The model under review builds one solid part; all positions refer to its coordinate system, in mm. Coordinates: 2 decimals unless noted, no trailing zeros. Loops run counter-clockwise (first coordinate to the right, second up) from the corner with the lowest first, then second, coordinate; pieces in that order, holes last. Notation, with made-up numbers: (-34.5, 10.5) - (-3.5, 10.5) arc R27 cw to (-3.5, 30.5) - close; hole circle Ø11 at (63.5, -24). An arc over 180 degrees is marked (long way). Answer in a Markdown table with one row per item. Add a question column.
(1) We need section A-A on y = -11.5. Write out the cut boundary in (x, z).
(2) For line 1 along Y through (x, z) = (54.5, 4.5); line 2 along Y through (x, z) = (72.5, 7.75); line 3 along Z through (x, y) = (94.65, 0), list the stretches that pass through material, from the lowest coordinate up.
(3) We need section B-B on z = 3.75. Write out the cut boundary in (x, y).
(4) We need section C-C on x = 46. Write out the cut boundary in (y, z).
(5) For P1, Ø1.5, axis at y = -10.5, z = 8.5, coming from the +X side; P2, Ø4.5, axis at y = 0, z = 3.75, coming from the +X side; P3, Ø1.5, axis at y = 0, z = 8.5, coming from the -X side; P4, Ø1.5, axis at x = 34.5, z = 8.5, coming from the +Y side, all flat-tipped, find the tip position at first contact; note any pin that passes through.
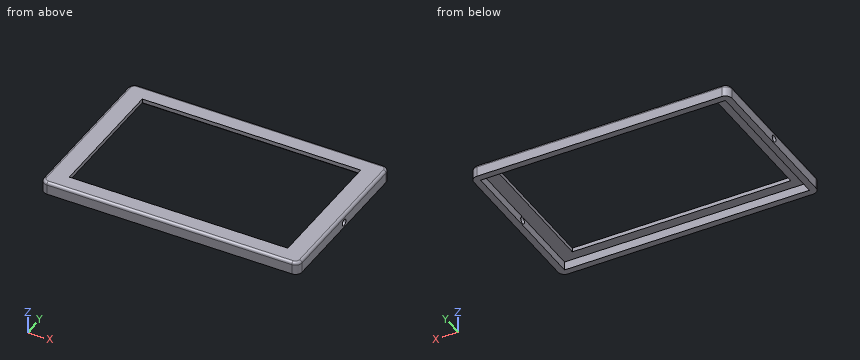
from build123d import *

# Parameters (mm, degrees)
SKETCH2_W           = 195
SKETCH2_H           = 125
SKETCH2_W_2         = 185
SKETCH2_H_2         = 115
BOSS_EXTRUDE1_DEPTH = 9.5
SKETCH3_W           = 195
SKETCH3_H           = 125
SKETCH3_W_2         = 165
SKETCH3_H_2         = 100
BOSS_EXTRUDE2_DEPTH = 3
FILLET1_R           = 5
FILLET2_R           = 2
SKETCH4_R           = 2.5
CUT_EXTRUDE1_DEPTH  = 205.991463237


with BuildPart() as part:
    # Sketch2 → Boss-Extrude1 (new body)
    with BuildSketch(Plane.XY):
        Rectangle(SKETCH2_W, SKETCH2_H)
        Rectangle(SKETCH2_W_2, SKETCH2_H_2, mode=Mode.SUBTRACT)
    extrude(amount=BOSS_EXTRUDE1_DEPTH)

    # Sketch3 → Boss-Extrude2 (add)
    with BuildSketch(Plane.XY.offset(9.5)):
        Rectangle(SKETCH3_W, SKETCH3_H)
        Rectangle(SKETCH3_W_2, SKETCH3_H_2, mode=Mode.SUBTRACT)
    extrude(amount=-BOSS_EXTRUDE2_DEPTH)

    # Fillet1
    fillet1_edges = [part.edges().sort_by_distance(p)[0] for p in [
        (-97.5, 62.5, 4.75),
        (97.5, 62.5, 4.75),
        (97.5, -62.5, 4.75),
        (-97.5, -62.5, 4.75),
    ]]
    fillet(fillet1_edges, radius=FILLET1_R)

    # Fillet2
    fillet2_edges = [part.edges().sort_by_distance(p)[0] for p in [
        (0, 62.5, 9.5),
        (-96.035533906, 61.035533906, 9.5),
        (96.035533906, 61.035533906, 9.5),
        (-97.5, 0, 9.5),
        (97.5, 0, 9.5),
        (-96.035533906, -61.035533906, 9.5),
        (96.035533906, -61.035533906, 9.5),
        (0, -62.5, 9.5),
    ]]
    fillet(fillet2_edges, radius=FILLET2_R)

    # Sketch4 → Cut-Extrude1 (cut, through all)
    with BuildSketch(Plane.ZY.offset(97.5)):
        with Locations(Location((3.75, 0, 0), (0, 0, 270))):
            Circle(SKETCH4_R)
    extrude(amount=-CUT_EXTRUDE1_DEPTH, mode=Mode.SUBTRACT)


solid = part.part
Outcome:
| question | item | result |
|---|---|---|
| 1 | outline | (-97.5, 0) - (-92.5, 0) - (-92.5, 6.5) - (-82.5, 6.5) - (-82.5, 9.5) - (-95.5, 9.5) arc R2 ccw to (-97.5, 7.5) - close; (82.5, 6.5) - (92.5, 6.5) - (92.5, 0) - (97.5, 0) - (97.5, 7.5) arc R2 ccw to (95.5, 9.5) - (82.5, 9.5) - close |
| 2 | line 1 | -62.5 to -57.5, 57.5 to 62.5 |
| 2 | line 2 | -62.48 to -50, 50 to 62.48 |
| 2 | line 3 | 0 to 1.25, 6.25 to 9.5 |
| 3 | outline | (-97.5, -57.5) arc R5 ccw to (-92.5, -62.5) - (92.5, -62.5) arc R5 ccw to (97.5, -57.5) - (97.5, -2.5) - (92.5, -2.5) - (92.5, -57.5) - (-92.5, -57.5) - (-92.5, -2.5) - (-97.5, -2.5) - close; (-97.5, 2.5) - (-92.5, 2.5) - (-92.5, 57.5) - (92.5, 57.5) - (92.5, 2.5) - (97.5, 2.5) - (97.5, 57.5) arc R5 ccw to (92.5, 62.5) - (-92.5, 62.5) arc R5 ccw to (-97.5, 57.5) - close |
| 4 | outline | (-62.5, 0) - (-57.5, 0) - (-57.5, 6.5) - (-50, 6.5) - (-50, 9.5) - (-60.5, 9.5) arc R2 ccw to (-62.5, 7.5) - close; (50, 6.5) - (57.5, 6.5) - (57.5, 0) - (62.5, 0) - (62.5, 7.5) arc R2 ccw to (60.5, 9.5) - (50, 9.5) - close |
| 5 | P1 | x = 97.48 |
| 5 | P2 | through |
| 5 | P3 | x = -97.48 |
| 5 | P4 | y = 62.48 |
